from build123d import *

# Parameters (mm, degrees)
F1_W      = 52.4
F1_H      = 72.4
F2_DEPTH  = 15
F3_T      = -1.2
F0_R      = 1
F4_DEPTH  = 10
F5_DEPTH  = 13
F6_R      = 1
F8_W      = 50.8
F8_H      = 70.8
F8_W_2    = 50
F8_H_2    = 70
F9_DEPTH  = 5
F10_W     = 10
F10_H     = 10
F11_DEPTH = 25


# Not quite as in the source:
# - two fillets or chamfers of one size are made in one step


with BuildPart() as f2:
    # F1 (on Top) → F2 (new body)
    with BuildSketch(Plane.XY):
        with Locations((25, 35)):
            Rectangle(F1_W, F1_H)
    extrude(amount=F2_DEPTH)

    # F3
    f3_openings = [f2.faces().sort_by_distance(p)[0] for p in [
        (25, 35, 15),
    ]]
    offset(amount=F3_T, openings=f3_openings)

    # F0 (on Top) → F4 (join)
    with BuildSketch(Plane.XY):
        with BuildLine():
            Line((4, 70), (0, 70))
            Line((0, 70), (0, 66))
            Line((0, 66), (3, 66))
            ThreePointArc((3, 66), (3.7071067812, 66.2928932188), (4, 67))
            Line((4, 67), (4, 70))
        make_face()
        with Locations((2, 68)):
            Circle(F0_R, mode=Mode.SUBTRACT)
        with BuildLine():
            Line((47, 66), (50, 66))
            Line((50, 66), (50, 70))
            Line((50, 70), (46, 70))
            Line((46, 70), (46, 67))
            ThreePointArc((46, 67), (46.2928932188, 66.2928932188), (47, 66))
        make_face()
        with Locations((48, 68)):
            Circle(F0_R, mode=Mode.SUBTRACT)
        with BuildLine():
            Line((50, 0), (50, 4))
            Line((50, 4), (47, 4))
            ThreePointArc((47, 4), (46.2928932188, 3.7071067812), (46, 3))
            Line((46, 3), (46, 0))
            Line((46, 0), (50, 0))
        make_face()
        with Locations((48, 2)):
            Circle(F0_R, mode=Mode.SUBTRACT)
        with BuildLine():
            ThreePointArc((4, 3), (3.7071067812, 3.7071067812), (3, 4))
            Line((3, 4), (0, 4))
            Line((0, 4), (0, 0))
            Line((0, 0), (4, 0))
            Line((4, 0), (4, 3))
        make_face()
        with Locations((2, 2)):
            Circle(F0_R, mode=Mode.SUBTRACT)
    extrude(amount=F4_DEPTH)

    # F5 (add): faces of the model
    f5_faces = [f2.faces().sort_by_distance(p)[0] for p in [
        (2, 2, 1.2),
        (48, 2, 1.2),
        (2, 68, 1.2),
        (48, 68, 1.2),
    ]]
    extrude(f5_faces, amount=F5_DEPTH)

    # F6
    f6_edges = [f2.edges().sort_by_distance(p)[0] for p in [
        (1, 2, 14.2),
        (47, 2, 14.2),
        (1, 68, 14.2),
        (47, 68, 14.2),
        (-1.2, -1.2, 7.5),
        (51.2, -1.2, 7.5),
        (-1.2, 71.2, 7.5),
        (51.2, 71.2, 7.5),
    ]]
    fillet(f6_edges, radius=F6_R)

    # F8 (on face) → F9 (cut)
    with BuildSketch(Plane.XY.offset(15)):
        with Locations((25, 35)):
            Rectangle(F8_W, F8_H)
        with Locations((25, 35)):
            Rectangle(F8_W_2, F8_H_2, mode=Mode.SUBTRACT)
    extrude(amount=-F9_DEPTH, mode=Mode.SUBTRACT)

    # F10 (on face) → F11 (cut)
    with BuildSketch(Plane.XZ.offset(1.2)):
        with Locations((25, 15)):
            Rectangle(F10_W, F10_H)
    extrude(amount=-F11_DEPTH, mode=Mode.SUBTRACT)


solid = f2.part
The listing builds one solid part. Answer for the finished solid, in the listing's coordinates (mm). A direction names the side the tool comes from. Coordinates: 2 decimals unless noted, no trailing zeros. Write each loop counter-clockwise with the first axis right and the second up, starting at its lowest first coordinate (ties: lowest second). Pieces come first, ordered by that corner, then holes. Notation, with made-up numbers: (-9, 78.5) - (12, 78.5) arc R13 cw to (12, 83.5) - close; hole circle Ø9 at (24, 67.25). An arc over 180 degrees is marked (long way). Put each result on its own line as item: value.
1. The part is cut by section A-A on x = 27. Give the vertices of the cut face in (y, z), plus the area to 3 significant figures.
Answer sheet:
outline: (-1.2, 0) - (71.2, 0) - (71.2, 15) - (70.4, 15) - (70.4, 10) - (70, 10) - (70, 1.2) - (0, 1.2) - (0, 10) - (-1.2, 10) - close
area: 112 mm^2
2. Determine the mould class of faces 1 (the face through (51.2, 35, 7)), 2 (the face through (50.4, 35, 13)), 3 (the face through (25, -1.2, 7)) for opening direction Y: pulls with the +Y half, pulls with the -Y half, needs draft (parallel to the pull), parting line crosses it, or undercut.
Answer sheet:
face 1: needs draft
face 2: undercut
face 3: pulls with the -Y half
3. A tool of negligible diameter and unlimited length cuts with its end or side. For faces 4 (the face through (40, -0.4, 13)), 5 (the face through (-1.2, 35, 7)), from which of +Z, -Z, +X, -X, +Y, -Y can it reach the whole face along a straight path? Write none if from no direction.
Answer sheet:
face 4: +Z
face 5: +Z, -Z, -X, +Y, -Y
4. The part is cut by section D-D on x = 8.5. Give the vertices of the cut face in (y, z), plus the area to 3 significant figures.
Answer sheet:
outline: (-1.2, 0) - (71.2, 0) - (71.2, 15) - (70.4, 15) - (70.4, 10) - (70, 10) - (70, 1.2) - (0, 1.2) - (0, 10) - (-0.4, 10) - (-0.4, 15) - (-1.2, 15) - close
area: 116 mm^2
5. The part is cut by section C-C on z = 8. Give the vertices of the cut face in (x, y).
Answer sheet:
outline: (-1.2, -0.2) arc R1 ccw to (-0.2, -1.2) - (50.2, -1.2) arc R1 ccw to (51.2, -0.2) - (51.2, 70.2) arc R1 ccw to (50.2, 71.2) - (-0.2, 71.2) arc R1 ccw to (-1.2, 70.2) - close; hole (0, 4) - (3, 4) arc R1 cw to (4, 3) - (4, 0) - (46, 0) - (46, 3) arc R1 cw to (47, 4) - (50, 4) - (50, 66) - (47, 66) arc R1 cw to (46, 67) - (46, 70) - (4, 70) - (4, 67) arc R1 cw to (3, 66) - (0, 66) - close
6. Find the intervals of material crossed by line 1 along X through (y, z) = (60.5, 9.5); line 2 along Y through (x, z) = (13, 12.5); line 3 along Y through (x, z) = (9.5, 8), in increasing order. Write a range as from..to.
Answer sheet:
line 1: x = -1.2..0, 50..51.2
line 2: y = -1.2..-0.4, 70.4..71.2
line 3: y = -1.2..0, 70..71.2
7. The part is cut by section B-B on y = 2. Give the vertices of the cut face in (x, z).
Answer sheet:
outline: (-1.2, 0) - (51.2, 0) - (51.2, 15) - (50.4, 15) - (50.4, 10) - (49, 10) - (49, 13.2) arc R1 ccw to (47, 13.2) - (47, 10) - (46, 10) - (46, 1.2) - (4, 1.2) - (4, 10) - (3, 10) - (3, 13.2) arc R1 ccw to (1, 13.2) - (1, 10) - (-0.4, 10) - (-0.4, 15) - (-1.2, 15) - close
8. Flat-ended cylindrical pins translate along their axes: pin 1 Ø1 at (x, y) = (25, 41) entering from +Z; pin 2 Ø1.5 at (x, z) = (23.5, 11.5) entering from -Y; pin 3 Ø0.9 at (y, z) = (-1, 11.5) entering from +X. Find the tip coordinate at first contact, or state that the pin passes through.
Answer sheet:
pin 1: stops at z = 1.2
pin 2: stops at y = 70.4
pin 3: stops at x = 51.14
